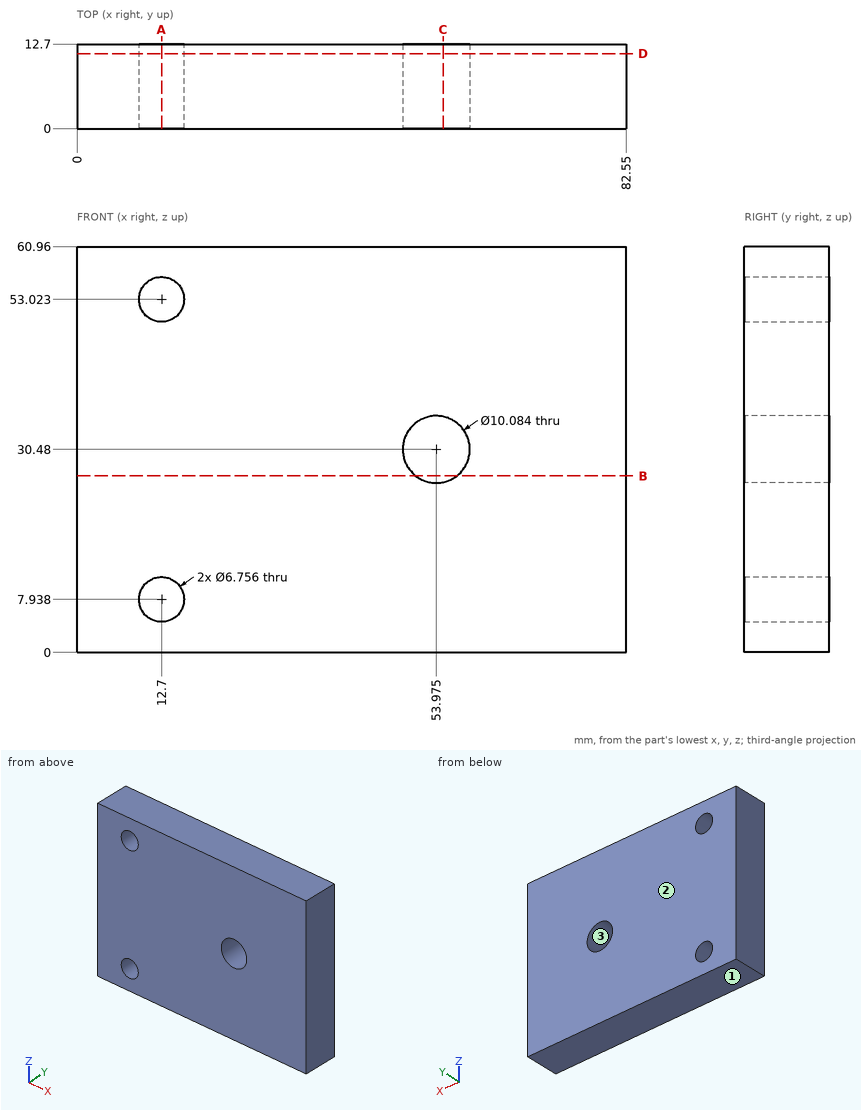
Could you check a few things on this drawing? It's one solid part, dimensions in mm from its lowest x, y, z. Round coordinates to 2 decimals unless told otherwise and drop trailing zeros. Order: outer loops, then holes, each group sorted by start corner. A loop starts at its lowest first (then second) coordinate and runs counter-clockwise, first axis right, second up. Notation, with made-up numbers: M 60,-26 L 83,-26 A25 cw 83,-6 Z; hole C 85,6 d4. An arc over 180 degrees is marked long. Return JSON: item names as keys, results as strings. Group by question number.
1. If we section it at A-A on x = 12.7: List the corners of the cut face in (y, z) for me (1 decimal).
2. If we mould it in two halves opening along Z, with no side actions, what happens to the marked faces 1, 2 and 3? For each: pulls with the +Z half, pulls with the -Z half, needs draft (parallel to the pull), parting line crosses it, or undercut.
3. Please list where these lines run through material, in increasing order: probe 1 along Z at (x, y) = (12.7, 8.75) (1 decimal); probe 2 along X at (y, z) = (11.5, 33); probe 3 along Z at (x, y) = (55, 12.25).
4. If we section it at B-B on z = 26.5: List the corners of the cut face in (x, y) for me, then the cut area to 3 significant figures.
5. If we section it at D-D on y = 11.25: State how many separate pieces and enclosed holes the cut face has, then the cut area to 3 significant figures.
6. If we section it at C-C on x = 55: List the corners of the cut face in (y, z) for me, then the cut area to 3 significant figures.
7. I'm going to push flat-ended pins straight in: pin 1 Ø5 at (x, z) = (30, 33.5) entering from -Y; pin 2 Ø5.5 at (x, z) = (12.7, 7.94) entering from -Y. Where does each tip first touch, or does it pass through?
Reply:
{
 "1": {"outline": "M 0,0 L 12.7,0 L 12.7,4.6 L 0,4.6 Z; M 0,11.3 L 12.7,11.3 L 12.7,49.6 L 0,49.6 Z; M 0,56.4 L 12.7,56.4 L 12.7,61 L 0,61 Z"},
 "2": {"face 1": "pulls with the -Z half", "face 2": "needs draft", "face 3": "undercut"},
 "3": {"probe 1": "0 to 4.6, 11.3 to 49.6, 56.4 to 61", "probe 2": "0 to 49.61, 58.34 to 82.55", "probe 3": "0 to 25.54, 35.42 to 60.96"},
 "4": {"outline": "M 0,0 L 50.88,0 L 50.88,12.7 L 0,12.7 Z; M 57.07,0 L 82.55,0 L 82.55,12.7 L 57.07,12.7 Z", "area": "970 mm^2"},
 "5": {"separate pieces": "1", "enclosed holes": "3", "area": "4,880 mm^2"},
 "6": {"outline": "M 0,0 L 12.7,0 L 12.7,25.54 L 0,25.54 Z; M 0,35.42 L 12.7,35.42 L 12.7,60.96 L 0,60.96 Z", "area": "649 mm^2"},
 "7": {"pin 1": "y = 0", "pin 2": "through"}
}
